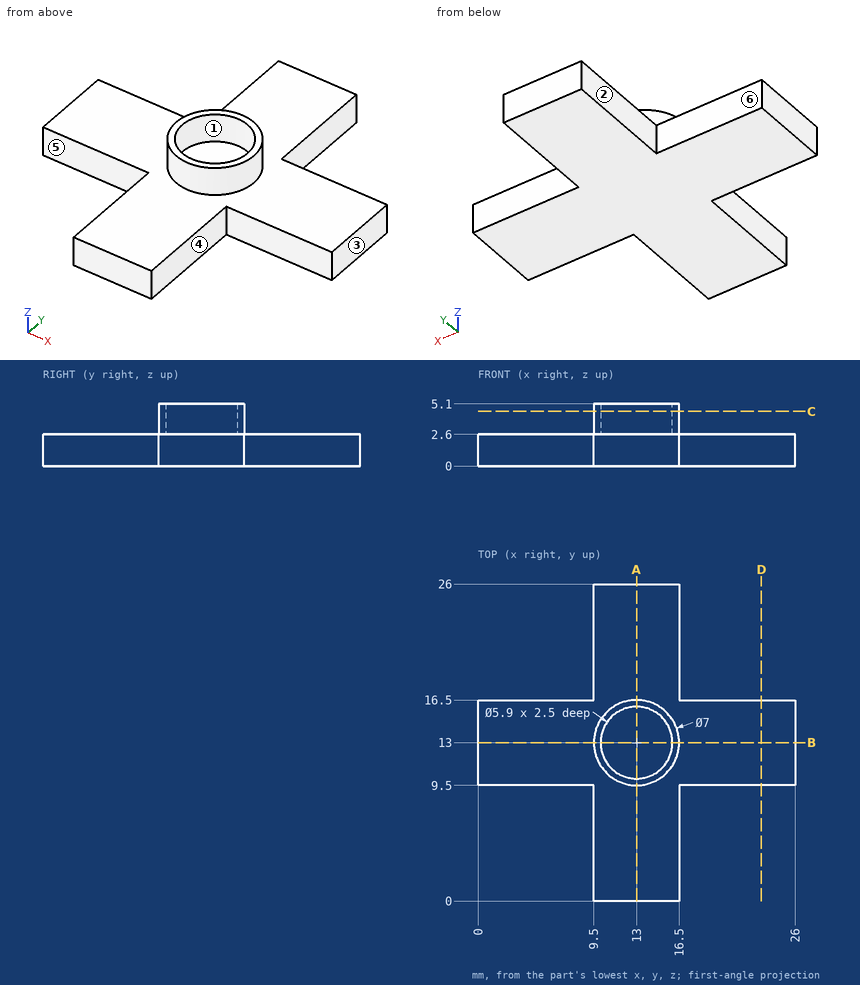
Geometry: see drawing. Coordinates: mm, zero at the bounding-box minimum. A direction names the side the tool comes from. Round coordinates to 2 decimals unless told otherwise and drop trailing zeros. Write each loop counter-clockwise with the first axis right and the second up, starting at its lowest first coordinate (ties: lowest second). Pieces come first, ordered by that corner, then holes.
Item 1: Section query D-D (x = 23.25). Return loops of the section in (y, z), plus the area to 3 significant figures.
Item 2: Pin query (flat end, axial travel): P1, Ø2, axis at y = 7, z = 2, coming from the -X side; P2, Ø4.5, axis at x = 13, y = 13, coming from the +Z side; P3, Ø2, axis at y = 4.5, z = 1.5, coming from the +X side. Return the tip coordinate at first contact, or that it passes through.
Item 3: Mould query, pull axis X, two halves, no side actions, for the marked faces 1, 2 and 3. Classes: +X half, -X half, draft (parallel to the pull), parting line (faces both ways), or undercut.
Item 4: Section query A-A (x = 13). Return loops of the section in (y, z).
Item 5: Material intervals for L1, parallel to Y at x = 13, z = 3.2; L2, parallel to Z at x = 16.5, y = 12.5; L3, parallel to Y at x = 7.5, z = 0.9, sorted ascending.
Item 6: Set-up query: the marked faces 4, 5 and 6. Return all of +Z, -Z, +X, -X, +Y, -Y with unobstructed straight access to the full face (end or side cutting, diameter ignored); none if empty.
Item 7: Section query C-C (z = 4.5). Return loops of the section in (x, y).
Completed:
1. outline: (9.5, 0) - (16.5, 0) - (16.5, 2.6) - (9.5, 2.6) - close
1. area: 18.2 mm2
2. P1: stops at x = 9.5
2. P2: stops at z = 2.6
2. P3: stops at x = 16.5
3. face 1: undercut
3. face 2: -X half
3. face 3: +X half
4. outline: (0, 0) - (26, 0) - (26, 2.6) - (16.5, 2.6) - (16.5, 5.1) - (15.95, 5.1) - (15.95, 2.6) - (10.05, 2.6) - (10.05, 5.1) - (9.5, 5.1) - (9.5, 2.6) - (0, 2.6) - close
5. L1: y = 9.5 to 10.05, 15.95 to 16.5
5. L2: z = 0 to 2.6
5. L3: y = 9.5 to 16.5
6. face 4: +Z, -Z, +X, -Y
6. face 5: +Z, -Z, -X, -Y
6. face 6: +Z, -Z, -X, +Y
7. outline: circle Ø7 at (13, 13); hole circle Ø5.9 at (13, 13)
